```python
from build123d import *

# Parameters (mm, degrees)
F1_DEPTH = 30


with BuildPart() as f1:
    # F0 (on Front) → F1 (new body)
    with BuildSketch(Plane.XZ):
        with BuildLine():
            Line((97.776912, 40.647307), (-80.380566, 40.647307))
            add(Edge.make_bspline(
                [(-80.380566, 40.647307), (-86.100639, 40.647307), (-86.100639, 40.647307), (-86.100639, 35.409246)],
                knots=[0, 0, 0, 0, 7.756063, 7.756063, 7.756063, 7.756063], degree=3))
            Line((-86.100639, 35.409246), (-86.100639, 23.107393))
            Line((-86.100639, 23.107393), (-86.100639, 13.742078))
            add(Edge.make_bspline(
                [(-86.100639, 13.742078), (-86.100639, 11.200923), (-84.778505, 9.990849), (-82.721377, 9.990849)],
                knots=[0, 0, 0, 0, 5.048874, 5.048874, 5.048874, 5.048874], degree=3))
            Line((-82.721377, 9.990849), (42.946892, 9.990849))
            Line((42.946892, 9.990849), (100.42418, 9.990849))
            add(Edge.make_bspline(
                [(100.42418, 9.990849), (100.899361, 10.444165), (100.899361, 11.027312), (100.899361, 11.835068)],
                knots=[0.810614, 0.810614, 0.810614, 0.810614, 2.726205, 2.726205, 2.726205, 2.726205], degree=3))
            Line((100.899361, 11.835068), (100.899361, 37.817217))
            Line((100.899361, 37.817217), (100.899361, 38.309757))
            add(Edge.make_bspline(
                [(97.776912, 40.647307), (98.709423, 40.647307), (100.746087, 40.282354), (100.899361, 38.309757)],
                knots=[0, 0, 0, 0, 3.908681, 3.908681, 3.908681, 3.908681], degree=3))
        make_face()
        with BuildLine():
            Line((42.946892, 9.990849), (-82.721377, 9.990849))
            Line((-82.721377, 9.990849), (-16.793105, 6.002678))
            Line((-16.793105, 6.002678), (-4.816184, 5.278163))
            Line((-4.816184, 5.278163), (22.046749, 3.653155))
            add(Edge.make_bspline(
                [(22.046749, 3.653155), (34.664334, 2.02508), (43.747929, 2.097842), (50.165818, -12.407815)],
                knots=[0, 0, 0, 0, 32.382662, 32.382662, 32.382662, 32.382662], degree=3))
            Line((50.165818, -12.407815), (42.946892, 9.990849))
        make_face()
        with BuildLine():
            add(Edge.make_bspline(
                [(99.762504, 9.572628), (100.049352, 9.699678), (100.263823, 9.837871), (100.42418, 9.990849)],
                knots=[0.164171, 0.164171, 0.164171, 0.164171, 0.810614, 0.810614, 0.810614, 0.810614], degree=3))
            Line((100.42418, 9.990849), (42.946892, 9.990849))
            Line((42.946892, 9.990849), (50.165818, -12.407815))
            Line((50.165818, -12.407815), (54.594625, -26.149378))
            Line((54.594625, -26.149378), (72.310335, -81.117139))
            add(Edge.make_bspline(
                [(72.310335, -81.117139), (73.538602, -84.92817), (76.174926, -86.352693), (79.634588, -86.352693)],
                knots=[0, 0, 0, 0, 9.003094, 9.003094, 9.003094, 9.003094], degree=3))
            Line((79.634588, -86.352693), (117.39595, -86.352693))
            add(Edge.make_bspline(
                [(126.196032, -81.440722), (126.605711, -86.352693), (122.000841, -86.352693), (117.39595, -86.352693)],
                knots=[0, 0, 0, 0, 10.07814, 10.07814, 10.07814, 10.07814], degree=3))
            add(Edge.make_bspline(
                [(99.529658, 9.477928), (74.162825, -1.021876), (121.11838, -42.338561), (126.196032, -81.440722)],
                knots=[1.614811, 1.614811, 1.614811, 1.614811, 95.760536, 95.760536, 95.760536, 95.760536], degree=3))
            add(Edge.make_bspline(
                [(99.762504, 9.572628), (99.684221, 9.541346), (99.606607, 9.509779), (99.529658, 9.477928)],
                knots=[1.329225, 1.329225, 1.329225, 1.329225, 1.614811, 1.614811, 1.614811, 1.614811], degree=3))
        make_face()
        with BuildLine():
            Line((-4.816184, 5.278163), (-16.793105, 6.002678))
            add(Edge.make_bspline(
                [(-16.793105, 6.002678), (-12.01583, 4.90427), (-12.169383, -16.80378), (-15.487377, -21.927638)],
                knots=[0, 0, 0, 0, 26.254366, 26.254366, 26.254366, 26.254366], degree=3))
            add(Edge.make_bspline(
                [(-15.487377, -21.927638), (-15.561956, -22.042808), (-15.638135, -22.1496), (-15.715892, -22.247591)],
                knots=[26.254366, 26.254366, 26.254366, 26.254366, 26.844495, 26.844495, 26.844495, 26.844495], degree=3))
            add(Edge.make_bspline(
                [(-15.715892, -22.247591), (-15.984637, -22.712274), (-15.798589, -22.976652), (-14.969375, -23.014201)],
                knots=[0.209384, 0.209384, 0.209384, 0.209384, 1.203722, 1.203722, 1.203722, 1.203722], degree=3))
            Line((-14.969375, -23.014201), (33.024817, -25.187522))
            add(Edge.make_bspline(
                [(33.024817, -25.187522), (35.429672, -25.345404), (36.811816, -25.272874), (38.675787, -24.702951)],
                knots=[0, 0, 0, 0, 5.671708, 5.671708, 5.671708, 5.671708], degree=3))
            add(Edge.make_bspline(
                [(38.675787, -24.702951), (42.706189, -22.769051), (51.420407, -20.362724), (54.594625, -26.149378)],
                knots=[1.903191, 1.903191, 1.903191, 1.903191, 17.202754, 17.202754, 17.202754, 17.202754], degree=3))
            Line((54.594625, -26.149378), (50.165818, -12.407815))
            add(Edge.make_bspline(
                [(34.029736, -21.737423), (37.275825, -21.454684), (52.078497, -18.342414), (50.165818, -12.407815)],
                knots=[0, 0, 0, 0, 18.639065, 18.639065, 18.639065, 18.639065], degree=3))
            Line((34.029736, -21.737423), (-4.816184, -19.978363))
            add(Edge.make_bspline(
                [(-4.816184, 5.278163), (-11.526522, 4.791767), (-12.252566, -21.466842), (-4.816184, -19.978363)],
                knots=[0, 0, 0, 0, 25.256526, 25.256526, 25.256526, 25.256526], degree=3))
        make_face()
    extrude(amount=F1_DEPTH)


solid = f1.part
```
Design review of the part built by this model. Coordinates are the model's own, in mm. A direction names the side the tool comes from. Coordinates: 2 decimals unless noted, no trailing zeros. Order: outer loops, then holes, each group sorted by start corner. A loop starts at its lowest first (then second) coordinate and runs counter-clockwise, first axis right, second up. Notation, with made-up numbers: (25.5, -13) - (44.5, -13) arc R28 cw to (44.5, 15) - close; hole circle Ø8 at (46.25, -38.75). An arc over 180 degrees is marked (long way). One line per question, with ' | ' between items.
Q1. Clearance check with flat-ended pins moving along their axes: pin 1 Ø8 at (x, y) = (-23.5, -8.5) entering from -Z; pin 2 Ø8 at (y, z) = (-8.5, 31.5) entering from +X; pin 3 Ø4 at (y, z) = (-11, 0) entering from -X. State where each tip first meets the part, or that it passes through.
Answer key:
pin 1: stops at z = 6.17 | pin 2: stops at x = 100.9 | pin 3: stops at x = -14.14
Q2. The part is to be moulded in two halves that separate along X. For faces 1 (the flat face through (8.427, -14.79, 4.477)), 2 (the flat face through (-86.101, -15, 25)), 3 (the flat face through (10, -15, 40.647)), say which applies: +X half, -X half, draft (parallel to the pull), parting line (faces both ways), or undercut.
Answer key:
face 1: undercut | face 2: -X half | face 3: draft
Q3. Consider section C-C, the plane x = 70. Give the boundary of the cut face in (y, z).
Answer key:
outline: (-30, -73.95) - (0, -73.95) - (0, 40.65) - (-30, 40.65) - close
Q4. Consider section B-B, the plane z = 19.5. Give the boundary of the cut face in (x, y), then the cut area to 3 significant figures.
Answer key:
outline: (-86.1, -30) - (100.9, -30) - (100.9, 0) - (-86.1, 0) - close | area: 5,610 mm2
Q5. Consider section A-A, the plane x = 19. Give the boundary of the cut face in (y, z), then the cut area to 3 significant figures.
Answer key:
outline: (-30, -24.55) - (0, -24.55) - (0, -21.06) - (-30, -21.06) - close; (-30, 3.84) - (0, 3.84) - (0, 40.65) - (-30, 40.65) - close | area: 1,210 mm2
Q6. For faces 4 (the flat face through (14.88, -14.79, -20.87)), 5 (the flat face through (42, -30, 6)), 6 (the flat face through (100.899, -15, 25)), list the 3-axis set-ups (+Z, -Z, +X, -X, +Y, -Y) from which the entire face can be reached by the end or side of a thin tool; tool diameter is ignored.
Answer key:
face 4: +Y, -Y | face 5: +Z, -Z, +X, -X, -Y | face 6: +Z, +X, +Y, -Y
Q7. To check wall thickness, follow line 1 along X through (y, z) = (-27, 20); line 2 along Z through (x, y) = (26, -9.5); line 3 along Z through (x, y) = (54, -23.5). State the ranges of each line that lie inside material, in increasing order.
Answer key:
line 1: x = -86.1 to 100.9 | line 2: z = -24.87 to -21.37, 3.17 to 40.65 | line 3: z = -25.24 to 40.65
